```python
from build123d import *

# Parameters (mm, degrees)
F0_W      = 212.6203179359
F0_H      = 22.2269091755
F1_DEPTH  = 25.4
F2_W      = 13.6859714985
F2_H      = 40.4146937653
F3_DEPTH  = 25.4
F5_DEPTH  = 25.4
F7_DEPTH  = 25.4
F8_W      = 86.2983710408
F8_H      = 107.4658855796
F9_DEPTH  = 25.4
F10_W     = 85.29484272
F10_H     = 40.7659783959
F11_DEPTH = 25.4
F12_W     = 86.2983710408
F12_H     = 148.2318639755
F13_DEPTH = 25.4
F15_W     = 73.2594318688
F15_H     = 64.30112198
F15_H_2   = 9.4412900507
F15_W_2   = 48.5810935497
F15_H_3   = 47.4680401385
F15_W_3   = 54.1693717241
F15_H_4   = 43.5468889773
F16_DEPTH = 25.4


with BuildPart() as f1:
    # F0 (on Front) → F1 (new body)
    with BuildSketch(Plane.XZ):
        Polygon((-136.7080956697, 70.86391747), (-136.7080956697, -9.9654700607), (75.9122222662, -9.9654700607), (78.8259357214, -9.9654700607), (78.8259357214, 70.86391747), align=None)
        with Locations((-30.3979367018, -21.0789246485)):
            Rectangle(F0_W, F0_H)
        Polygon((75.9122222662, -32.1923792362), (-136.7080956697, -32.1923792362), (-136.7080956697, -77.3679465055), (77.8233259916, -77.3679465055), (77.8233259916, -32.1923792362), align=None)
    extrude(amount=F1_DEPTH)

    # F2 (on face) → F3 (join)
    with BuildSketch(Plane.YZ.offset(78.8259357214)):
        Polygon((0, 30.4492237046), (0, 70.86391747), (-25.4, 70.86391747), (-25.4, -75.8049190044), (0, -75.8049190044), (0, -9.9654700607), (-13.6859714985, -9.9654700607), (-13.6859714985, 30.4492237046), align=None)
        with Locations((-6.8429857492, 10.241876822)):
            Rectangle(F2_W, F2_H)
    extrude(amount=F3_DEPTH)

    # F4 (on face) → F5 (join)
    with BuildSketch(Plane(origin=(0, 0, 0), x_dir=(-1, 0, 0), z_dir=(0, 1, 0))):
        Polygon((75.8066177368, -40.0540344417), (75.8066177368, -77.3679465055), (136.7080956697, -77.3679465055), (136.7080956697, 70.86391747), (75.8066177368, 70.86391747), (75.8066177368, 35.8203239739), (99.0835726261, 35.8203239739), (99.0835726261, -40.0540344417), align=None)
        Polygon((-17.9275646806, -77.3679465055), (75.8066177368, -77.3679465055), (75.8066177368, -40.0540344417), (24.7398540378, -40.0540344417), (24.7398540378, 35.8203239739), (75.8066177368, 35.8203239739), (75.8066177368, 70.86391747), (-17.9275646806, 70.86391747), align=None)
    extrude(amount=F5_DEPTH)

    # F6 (on face) → F7 (join)
    with BuildSketch(Plane(origin=(0, 25.4, 0), x_dir=(-1, 0, 0), z_dir=(0, 1, 0))):
        Polygon((24.7398540378, -40.0540344417), (24.7398540378, 14.7684887052), (-17.9275646806, 14.7684887052), (-17.9275646806, -77.3679465055), (77.9451653361, -77.3679465055), (77.9451653361, -40.0540344417), align=None)
        Polygon((-17.9275646806, 14.7684887052), (24.7398540378, 14.7684887052), (24.7398540378, 35.8203239739), (77.9451653361, 35.8203239739), (77.9451653361, 70.86391747), (-17.9275646806, 70.86391747), align=None)
        Polygon((77.9451653361, 70.86391747), (77.9451653361, 35.8203239739), (99.0835726261, 35.8203239739), (99.0835726261, -40.0540344417), (77.9451653361, -40.0540344417), (77.9451653361, -77.3679465055), (136.7080956697, -77.3679465055), (136.7080956697, 70.86391747), align=None)
    extrude(amount=F7_DEPTH)

    # F8 (on face) → F9 (join)
    with BuildSketch(Plane(origin=(0, 0, 0), x_dir=(-1, 0, 0), z_dir=(0, 1, 0))):
        with Locations((-61.076750201, 17.1309746802)):
            Rectangle(F8_W, F8_H)
    extrude(amount=F9_DEPTH)

    # F10 (on face) → F11 (join)
    with BuildSketch(Plane(origin=(0, 0, 0), x_dir=(-1, 0, 0), z_dir=(0, 1, 0))):
        with Locations((-60.5749860406, -56.9849573076)):
            Rectangle(F10_W, F10_H)
    extrude(amount=F11_DEPTH)

    # F12 (on face) → F13 (join)
    with BuildSketch(Plane(origin=(0, 25.4, 0), x_dir=(-1, 0, 0), z_dir=(0, 1, 0))):
        with Locations((-61.076750201, -3.2520145178)):
            Rectangle(F12_W, F12_H)
    extrude(amount=F13_DEPTH)

    # F15 (on face) → F16 (join)
    with BuildSketch(Plane(origin=(0, 50.8, 0), x_dir=(-1, 0, 0), z_dir=(0, 1, 0))):
        Polygon((25.0786952674, -29.877435416), (25.0786952674, 34.423686564), (98.3381271362, 34.423686564), (98.3381271362, -29.877435416), (135.9246820211, -29.877435416), (135.9246820211, 117.3784919083), (-83.4680050611, 117.3784919083), (-83.4680050611, 73.831602931), (-83.4680050611, 62.8992691636), (-83.4680050611, 15.4312290251), (-83.4680050611, -29.877435416), align=None)
        with Locations((61.7084112018, 2.273125574)):
            Rectangle(F15_W, F15_H)
        with Locations((61.7084112018, -34.5980804414)):
            Rectangle(F15_W, F15_H_2)
        with Locations((-107.758551836, 39.1652490944)):
            Rectangle(F15_W_2, F15_H_3)
        Polygon((-132.0490986109, 62.8992691636), (-83.4680050611, 62.8992691636), (-83.4680050611, 73.831602931), (-137.6373767853, 73.831602931), (-137.6373767853, 62.8992691636), align=None)
        with Locations((-110.5526909232, 95.6050474197)):
            Rectangle(F15_W_3, F15_H_4)
    extrude(amount=F16_DEPTH)


solid = f1.part
```
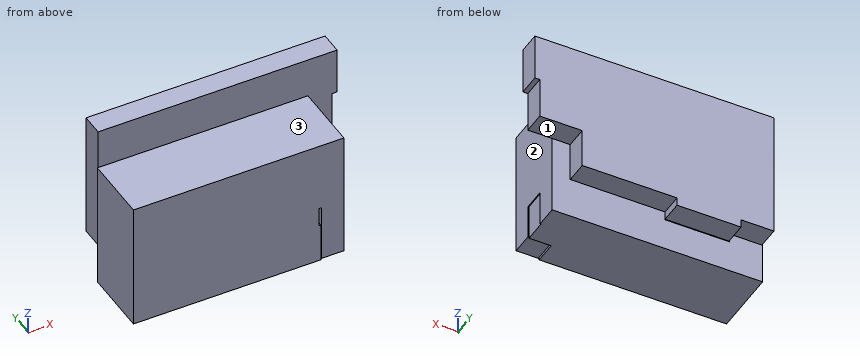
Source: CAD feature listing. Evaluate the final solid. Frame: model axes, mm. Face numbers are marked on the shaded views. A direction names the side the tool comes from. Give positions to 0.01 mm unless a question says otherwise; leave off trailing zeros. Order: outer loops, then holes, each group sorted by start corner. A loop starts at its lowest first (then second) coordinate and runs counter-clockwise, first axis right, second up.
(1) Access query for the marked faces 1, 2 and 3. Directions: +Z, -Z, +X, -X, +Y, -Y. A direction counts if a zero-diameter tool reaches every point of the face in a straight line with its end or side. Return the directions, or none.
(2) Section query B-B (z = 4). Return the cut outline in (x, y).
(3) Contact query for flat-ended pins moving along their axis: P1, Ø0.6, axis at x = 77, y = -10, coming from the +Z side; P2, Ø18, axis at y = -17, z = -17, coming from the +X side; P3, Ø4, axis at y = 55.5, z = -20.5, coming from the -X side. Output: stop coordinate, or through.
(4) Material intervals for line 1 along X through (y, z) = (15, -7); line 2 along Y through (x, z) = (-64, 5); line 3 along X through (y, z) = (-20, -53.5), sorted ascending.
(5) Section query C-C (x = 53). Return the cut outline in (y, z), plus the area to 3 significant figures.
(6) Section query A-A (y = 47). Return the cut outline in (x, z).
(7) Section query D-D (y = -13.5). Return the cut outline in (x, z).
Outcome:
1. face 1: -Z, +X, +Y
1. face 2: +Z, -Z, +X, -Y
1. face 3: +Z, +X, -X, -Y
2. outline: (-136.71, -25.4) - (104.23, -25.4) - (104.23, 50.8) - (83.47, 50.8) - (83.47, 76.2) - (-135.92, 76.2) - (-135.92, 50.8) - (-136.71, 50.8) - close; hole (-99.08, 0) - (-24.74, 0) - (-24.74, 50.8) - (-99.08, 50.8) - close
3. P1: stops at z = 70.86
3. P2: stops at x = 104.23
3. P3: stops at x = -135.92
4. line 1: x = -136.71 to -99.08, -24.74 to 104.23
4. line 2: y = -25.4 to 0, 50.8 to 76.2
4. line 3: x = -136.71 to 77.82, 78.83 to 104.23
5. outline: (-25.4, -77.37) - (50.8, -77.37) - (50.8, -29.88) - (76.2, -29.88) - (76.2, 117.38) - (50.8, 117.38) - (50.8, 70.86) - (-25.4, 70.86) - close
5. area: 15,000 mm2
6. outline: (-136.71, -77.37) - (104.23, -77.37) - (104.23, 70.86) - (-136.71, 70.86) - close; hole (-99.08, -40.05) - (-24.74, -40.05) - (-24.74, 35.82) - (-99.08, 35.82) - close
7. outline: (-136.71, -77.37) - (77.82, -77.37) - (77.82, -32.19) - (75.91, -32.19) - (75.91, -9.97) - (78.83, -9.97) - (78.83, -75.8) - (104.23, -75.8) - (104.23, 70.86) - (-136.71, 70.86) - close
